The listing builds one solid part. Answer for the finished solid, in the listing's coordinates (mm). A direction names the side the tool comes from. Round coordinates to 2 decimals unless told otherwise and drop trailing zeros. Write each loop counter-clockwise with the first axis right and the second up, starting at its lowest first coordinate (ties: lowest second). Pieces come first, ordered by that corner, then holes. Notation, with made-up numbers: (-23.5, -39) - (13.5, -39) arc R17 ccw to (13.5, -32) - close; hole circle Ø6 at (85.25, 79.25). An arc over 180 degrees is marked (long way). Return JSON: item names as keys, results as strings. Group by question number.
(1) Section B-B, the plane x = 19 is taken. Write down the section's boundary in (y, z) (3 decimals), then the cut area to 3 significant figures.
(2) Find the intervals of material crossed by line 1 along X through (y, z) = (-18, -0.05); line 2 along Y through (x, z) = (8.5, 0.4); line 3 along Y through (x, z) = (-10.5, -0.2), in increasing order. Write a range as [from, to].
(3) Section D-D, the plane x = 0 is taken. Write down the section's boundary in (y, z) (3 decimals).
(4) Determine the mould class of faces 1 (the cylindrical face through (-0.925, 24.232, -0.012)), 2 (the cylindrical face through (0.67, 19.94, -0.01)), 3 (the flat face through (4, 20, -0.875)) for opening direction Y: +Y half, -Y half, draft (parallel to the pull), parting line (faces both ways), or undercut.
(5) Which of the six approach directions +Z, -Z, +X, -X, +Y, -Y give full straight-line access (tool end or side, diameter ignored) to faces 4 (the flat face through (4, 20, 0.875)), 5 (the cylindrical face through (13.838, -16.256, -0.012)), 6 (the flat face through (-8.14, -20.19, -0.01))?
(6) Section A-A, the plane y = -11 is taken. Write down the section's boundary in (x, z) (1 decimal), then the cut area to 3 significant figures.
(7) Section C-C, the plane z = -0.45 is taken. Give the number of separate pieces and of enclosed holes in the cut face, then the cut area to 3 significant figures.
```python
from build123d import *

# Parameters (mm, degrees)
BOSS_EXTRUDE1_DEPTH      = 0.875
BOSS_EXTRUDE1_DEPTH_BACK = 0.875
SKETCH3_R                = 1.25
FILLET1_R                = 0.79375


with BuildPart() as part:
    # Sketch3 → Boss-Extrude1 (new, two sides: drawn at the far end of the back side and taken through both)
    with BuildSketch(Plane.XY.offset(-BOSS_EXTRUDE1_DEPTH_BACK)):
        with BuildLine():
            Line((-7.536269642, -18.690362219), (-9.068559557, -22.490525284))
            ThreePointArc((-9.068559557, -22.490525284), (0, 24.25), (9.068559557, -22.490525284))
            Line((9.068559557, -22.490525284), (7.536269642, -18.690362219))
            ThreePointArc((7.536269642, -18.690362219), (8.084526994, -16.229043526), (10.57907226, -15.860370565))
            ThreePointArc((10.57907226, -15.860370565), (13.884078483, -16.245316894), (16.696841294, -14.467786253))
            ThreePointArc((16.696841294, -14.467786253), (0, 19.95), (-16.696841294, -14.467786253))
            ThreePointArc((-16.696841294, -14.467786253), (-13.884078483, -16.245316894), (-10.57907226, -15.860370565))
            ThreePointArc((-10.57907226, -15.860370565), (-8.084526994, -16.229043526), (-7.536269642, -18.690362219))
        make_face()
        with Locations((-9.599833302, -17.858298507)):
            Circle(SKETCH3_R, mode=Mode.SUBTRACT)
        with Locations(Location((9.599833302, -17.858298507, 0), (0, 0, 180))):
            Circle(SKETCH3_R, mode=Mode.SUBTRACT)
    extrude(amount=BOSS_EXTRUDE1_DEPTH + BOSS_EXTRUDE1_DEPTH_BACK)

    # Fillet1
    fillet1_edges = [part.edges().sort_by_distance(p)[0] for p in [
        (9.068559557, -22.490525284, 0),
        (-9.068559557, -22.490525284, 0),
    ]]
    fillet(fillet1_edges, radius=FILLET1_R)


solid = part.part
```
Working result:
{
 "1": {"outline": "(-15.069, -0.875) - (-10.845, -0.875) - (-10.845, 0.875) - (-15.069, 0.875) - close; (8.227, -0.875) - (15.069, -0.875) - (15.069, 0.875) - (8.227, 0.875) - close", "area": "19.4 mm^2"},
 "2": {"line 1": "x = [-16.25, -10.84], [-8.36, -7.38], [7.38, 8.36], [10.84, 16.25]", "line 2": "y = [-21.08, -18.45], [-17.26, -15.92], [18.18, 22.71]", "line 3": "y = [-21.86, -18.73], [-16.99, -15.82], [17.18, 21.86]"},
 "3": {"outline": "(19.95, -0.875) - (24.25, -0.875) - (24.25, 0.875) - (19.95, 0.875) - close"},
 "4": {"face 1": "parting line", "face 2": "undercut", "face 3": "draft"},
 "5": {"face 4": "+Z, +X, -X, +Y, -Y", "face 5": "+Z, -Z", "face 6": "+Z, -Z, -Y"},
 "6": {"outline": "(-21.6, -0.9) - (-18.9, -0.9) - (-18.9, 0.9) - (-21.6, 0.9) - close; (18.9, -0.9) - (21.6, -0.9) - (21.6, 0.9) - (18.9, 0.9) - close", "area": "9.42 mm^2"},
 "7": {"separate pieces": "1", "enclosed holes": "2", "area": "431 mm^2"}
}
